Source: three-view drawing plus pictorial views. Frame: mm from the lowest corner of the part. Give positions to 0.01 mm unless a question says otherwise; leave off trailing zeros. Write each loop counter-clockwise with the first axis right and the second up, starting at its lowest first coordinate (ties: lowest second). Pieces come first, ordered by that corner, then holes. Notation, with made-up numbers: M 87.25,18 L 98.25,18 A17 ccw 98.25,34 Z; hole C 59,56.5 d4. An arc over 180 degrees is marked long. Return JSON: item names as keys, results as strings.
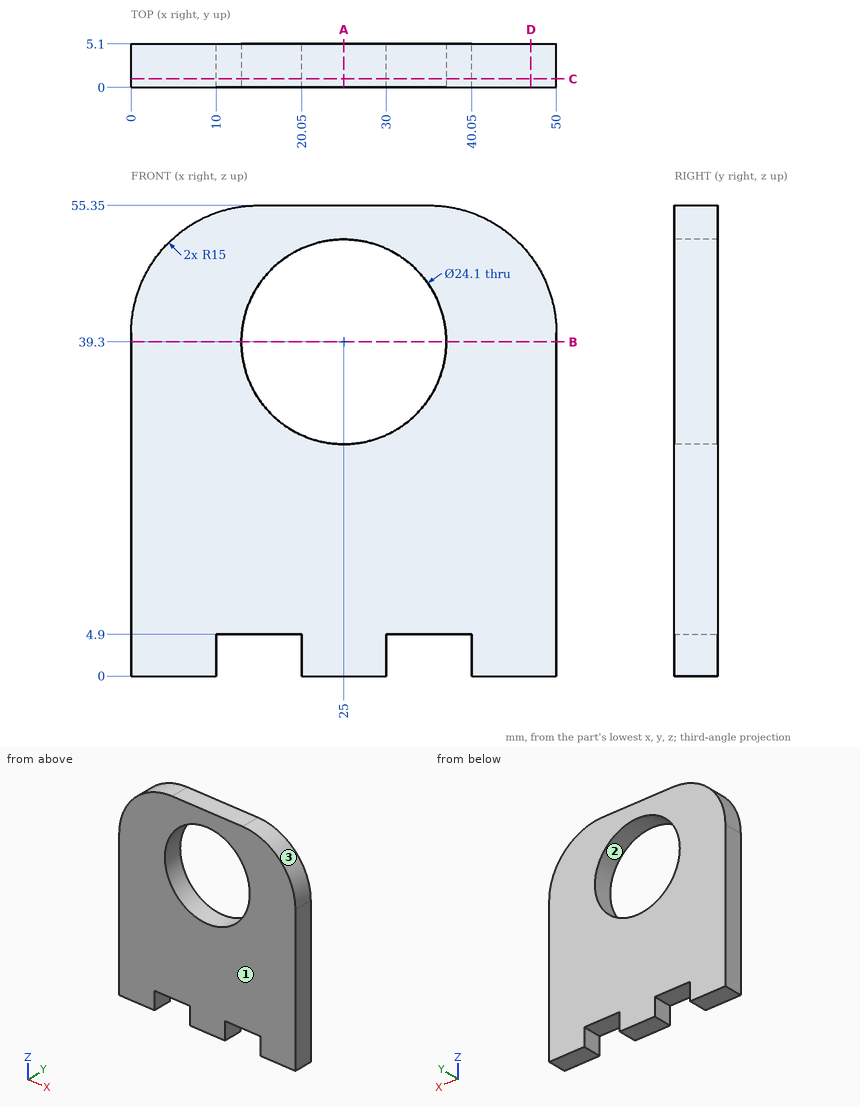
1) Cut plane D-D, the plane x = 47. Return the cut outline in (y, z), then the cut area to 3 significant figures.
Numbers:
{"outline": "M 0,0 L 5.1,0 L 5.1,49.35 L 0,49.35 Z", "area": "252 mm²"}
2) Cut plane B-B, the plane z = 39.3. Return the cut outline in (x, y).
Numbers:
{"outline": "M 0,0 L 12.95,0 L 12.95,5.1 L 0,5.1 Z; M 37.05,0 L 50,0 L 50,5.1 L 37.05,5.1 Z"}
3) Cut plane C-C, the plane y = 1. Return the cut outline in (x, z).
Numbers:
{"outline": "M 0,0 L 10,0 L 10,4.9 L 20.05,4.9 L 20.05,0 L 30,0 L 30,4.9 L 40.05,4.9 L 40.05,0 L 50,0 L 50,40.35 A15 ccw 35,55.35 L 15,55.35 A15 ccw 0,40.35 Z; hole C 25,39.3 d24.1"}
4) Contact query for flat-ended pins moving along their axis: pin 1 Ø1.5 at (x, y) = (18, 0.5) entering from -Z; pin 2 Ø21.5 at (x, z) = (25, 39.3) entering from +Y. Output: stop coordinate, or through.
Numbers:
{"pin 1": "stops at z = 4.9", "pin 2": "passes through"}
5) Draft query along X for the marked faces 1, 2 and 3. Return one class per face: released by +X, released by -X, zero draft, split by the parting line, or undercut.
Numbers:
{"face 1": "zero draft", "face 2": "undercut", "face 3": "released by +X"}
6) Cut plane A-A, the plane x = 25. Return the cut outline in (y, z), then the cut area to 3 significant figures.
Numbers:
{"outline": "M 0,0 L 5.1,0 L 5.1,27.25 L 0,27.25 Z; M 0,51.35 L 5.1,51.35 L 5.1,55.35 L 0,55.35 Z", "area": "159 mm²"}
7) Line query: line 1 (X direction, y = 2.9, z = 39.3); line 2 (Z direction, x = 25, y = 1.55); line 3 (X direction, y = 3, z = 44.5). Output: solid intervals per line, ascending. Write a range as [from, to].
Numbers:
{"line 1": "x = [0, 12.95], [37.05, 50]", "line 2": "z = [0, 27.25], [51.35, 55.35]", "line 3": "x = [0.59, 14.13], [35.87, 49.41]"}
